Model file for the job. Use its own axes, mm. A direction names the side the tool comes from. Give positions to 0.01 mm unless a question says otherwise; leave off trailing zeros. Write each loop counter-clockwise with the first axis right and the second up, starting at its lowest first coordinate (ties: lowest second). Pieces come first, ordered by that corner, then holes. Notation, with made-up numbers: M 61.25,-7 L 105.25,-7 A19 cw 105.25,12 Z; hole C 44.5,21.25 d10. An arc over 180 degrees is marked long. Answer as a JSON object with one key per item and string values. Group by question number.
```python
from build123d import *

# Parameters (mm, degrees)
F0_W     = 4.191
F0_H     = 9.4390108662
F0_W_2   = 2.159
F0_H_2   = 7.366
F0_W_3   = 0.889
F0_H_3   = 6.35
F1_DEPTH = 1.016
F2_DEPTH = 12.954


with BuildPart() as f1:
    # F0 (on Front) → F1 (new body)
    with BuildSketch(Plane.XZ):
        Polygon((-8.4455, 12.408932417), (-12.7, 12.408932417), (-12.7, -11.467067583), (12.7, -11.467067583), (12.7, 12.408932417), (0, 12.408932417), align=None)
        Polygon((-6.35, 9.9099432833), (-6.35, 0.470932417), (-6.35, -8.9680784492), (-10.541, -8.9680784492), (-10.541, 0.470932417), (-10.541, 9.9099432833), align=None, mode=Mode.SUBTRACT)
        Polygon((-2.0955, -8.9680784492), (-2.0955, 0.470932417), (-2.0955, 9.9099432833), (2.0955, 9.9099432833), (2.0955, 0.470932417), (2.0955, -8.9680784492), align=None, mode=Mode.SUBTRACT)
        Polygon((6.35, -8.9680784492), (6.35, 0.470932417), (6.35, 9.9099432833), (10.541, 9.9099432833), (10.541, 0.470932417), (10.541, -8.9680784492), align=None, mode=Mode.SUBTRACT)
        with Locations((-8.4455, 5.1904378501)):
            Rectangle(F0_W, F0_H)
        with Locations((-8.4455, 5.804932417)):
            Rectangle(F0_W_2, F0_H_2, mode=Mode.SUBTRACT)
        with Locations((-8.4455, 5.804932417)):
            Rectangle(F0_W_2, F0_H_2)
        with Locations((-8.4455, 5.804932417)):
            Rectangle(F0_W_3, F0_H_3, mode=Mode.SUBTRACT)
        with Locations((0, 5.1904378501)):
            Rectangle(F0_W, F0_H)
        with Locations((0, 5.804932417)):
            Rectangle(F0_W_2, F0_H_2, mode=Mode.SUBTRACT)
        with Locations((0, 5.804932417)):
            Rectangle(F0_W_2, F0_H_2)
        with Locations((0, 5.804932417)):
            Rectangle(F0_W_3, F0_H_3, mode=Mode.SUBTRACT)
        with Locations((0, -4.2485730161)):
            Rectangle(F0_W, F0_H)
        with Locations((0, -4.863067583)):
            Rectangle(F0_W_2, F0_H_2, mode=Mode.SUBTRACT)
        with Locations((0, -4.863067583)):
            Rectangle(F0_W_2, F0_H_2)
        with Locations((0, -4.863067583)):
            Rectangle(F0_W_3, F0_H_3, mode=Mode.SUBTRACT)
        with Locations((-8.4455, -4.2485730161)):
            Rectangle(F0_W, F0_H)
        with Locations((-8.4455, -4.863067583)):
            Rectangle(F0_W_2, F0_H_2, mode=Mode.SUBTRACT)
        with Locations((-8.4455, -4.863067583)):
            Rectangle(F0_W_2, F0_H_2)
        with Locations((-8.4455, -4.863067583)):
            Rectangle(F0_W_3, F0_H_3, mode=Mode.SUBTRACT)
        with Locations((8.4455, -4.2485730161)):
            Rectangle(F0_W, F0_H)
        with Locations((8.4455, -4.863067583)):
            Rectangle(F0_W_2, F0_H_2, mode=Mode.SUBTRACT)
        with Locations((8.4455, -4.863067583)):
            Rectangle(F0_W_2, F0_H_2)
        with Locations((8.4455, -4.863067583)):
            Rectangle(F0_W_3, F0_H_3, mode=Mode.SUBTRACT)
        with Locations((8.4455, 5.1904378501)):
            Rectangle(F0_W, F0_H)
        with Locations((8.4455, 5.804932417)):
            Rectangle(F0_W_2, F0_H_2, mode=Mode.SUBTRACT)
        with Locations((8.4455, 5.804932417)):
            Rectangle(F0_W_2, F0_H_2)
        with Locations((8.4455, 5.804932417)):
            Rectangle(F0_W_3, F0_H_3, mode=Mode.SUBTRACT)
    extrude(amount=-F1_DEPTH)

    # F0 (on Front) → F2 (join)
    with BuildSketch(Plane.XZ):
        with Locations((-8.4455, 5.1904378501)):
            Rectangle(F0_W, F0_H)
        with Locations((-8.4455, 5.804932417)):
            Rectangle(F0_W_2, F0_H_2, mode=Mode.SUBTRACT)
        with Locations((-8.4455, -4.2485730161)):
            Rectangle(F0_W, F0_H)
        with Locations((-8.4455, -4.863067583)):
            Rectangle(F0_W_2, F0_H_2, mode=Mode.SUBTRACT)
        with Locations((0, 5.1904378501)):
            Rectangle(F0_W, F0_H)
        with Locations((0, 5.804932417)):
            Rectangle(F0_W_2, F0_H_2, mode=Mode.SUBTRACT)
        with Locations((0, -4.2485730161)):
            Rectangle(F0_W, F0_H)
        with Locations((0, -4.863067583)):
            Rectangle(F0_W_2, F0_H_2, mode=Mode.SUBTRACT)
        with Locations((8.4455, 5.1904378501)):
            Rectangle(F0_W, F0_H)
        with Locations((8.4455, 5.804932417)):
            Rectangle(F0_W_2, F0_H_2, mode=Mode.SUBTRACT)
        with Locations((8.4455, -4.2485730161)):
            Rectangle(F0_W, F0_H)
        with Locations((8.4455, -4.863067583)):
            Rectangle(F0_W_2, F0_H_2, mode=Mode.SUBTRACT)
    extrude(amount=-F2_DEPTH)


solid = f1.part
```
Q1. Slice it at B-B, the plane z = 1.5. Write the cut outline in (x, y), then the cut area to 3 significant figures.
Q2. Wall check: L1, parallel to Z at x = -7.75, y = 5; L2, parallel to X at y = 7, z = -0.5; L3, parallel to X at y = 0.5, z = -8. Give the ranges that are in metal, low to high.
Q3. Two-plate mould, pull along Z, no slides. Class faces 1 (the flat face through (6.35, 7, 1)), 2 (the flat face through (-8, 7, 9.91)), 3 (the flat face through (-8.001, 0.5, -4.9)): +Z half, -Z half, draft (parallel to the pull), parting line (faces both ways), or undercut.
Q4. Slice it at A-A, the plane y = 1.5. Count the separate pieces of the cut face and the enclosed holes in it, then the cut area to 3 significant figures.
Q5. Slice it at C-C, the plane x = 2.5. Write the cut outline in (y, z), then the cut area to 3 significant figures.
Q6. Drop flat-ended pins along their axis: P1, Ø1.7, axis at x = -8.5, y = 8.5, coming from the -Z side; P2, Ø1, axis at x = 9, y = 2.5, coming from the +Z side; P3, Ø6, axis at y = 9.5, z = -5.5, coming from the -X side; P4, Ø12, axis at x = -6, z = -4, coming from the +Y side. Give the stop position or say it passes through.
Q7. 3-axis set-ups, long thin cutter, end or side, ignore diameter. For faces 4 (the flat face through (10.541, 7, 0)), 5 (the flat face through (0, 0.5, 2.63)), 6 (the flat face through (-8, 7, 2.122)): which of +Z, -Z, +X, -X, +Y, -Y reach the whole face in a straight line?
Solved:
{
 "1": {"outline": "M -12.7,0 L 12.7,0 L 12.7,1.02 L 10.54,1.02 L 10.54,12.95 L 6.35,12.95 L 6.35,1.02 L 2.1,1.02 L 2.1,12.95 L -2.1,12.95 L -2.1,1.02 L -6.35,1.02 L -6.35,12.95 L -10.54,12.95 L -10.54,1.02 L -12.7,1.02 Z", "area": "176 mm²"},
 "2": {"L1": "z = -8.97 to -8.55, -1.18 to 2.12, 9.49 to 9.91", "L2": "x = -10.54 to -6.35, -2.1 to 2.1, 6.35 to 10.54", "L3": "x = -12.7 to -8.89, -8 to -0.44, 0.44 to 8, 8.89 to 12.7"},
 "3": {"face 1": "draft", "face 2": "+Z half", "face 3": "undercut"},
 "4": {"separate pieces": "3", "enclosed holes": "6", "area": "142 mm²"},
 "5": {"outline": "M 0,-11.47 L 1.02,-11.47 L 1.02,12.41 L 0,12.41 Z", "area": "24.3 mm²"},
 "6": {"P1": "stops at z = -8.97", "P2": "stops at z = 9.91", "P3": "stops at x = -10.54", "P4": "stops at y = 12.95"},
 "7": {"face 4": "+Z, -Z, +X, +Y", "face 5": "+Y, -Y", "face 6": "+Y"}
}
